```python
from build123d import *

# Parameters (mm, degrees)
SKETCH1_W           = 165
SKETCH1_H           = 81
SKETCH1_W_2         = 74
SKETCH1_H_2         = 50
BOSS_EXTRUDE1_DEPTH = 6
SKETCH2_W           = 108
SKETCH2_H           = 68
SKETCH2_W_2         = 98.5
SKETCH2_H_2         = 58.5
BOSS_EXTRUDE2_DEPTH = 9


with BuildPart() as part:
    # Sketch1 → Boss-Extrude1 (new body)
    with BuildSketch(Plane.XY):
        Rectangle(SKETCH1_W, SKETCH1_H)
        Rectangle(SKETCH1_W_2, SKETCH1_H_2, mode=Mode.SUBTRACT)
    extrude(amount=BOSS_EXTRUDE1_DEPTH)

    # Sketch2 → Boss-Extrude2 (add)
    with BuildSketch(Plane.XY):
        Rectangle(SKETCH2_W, SKETCH2_H)
        Rectangle(SKETCH2_W_2, SKETCH2_H_2, mode=Mode.SUBTRACT)
    extrude(amount=BOSS_EXTRUDE2_DEPTH)


solid = part.part
```
The listing builds one solid part. Answer for the finished solid, in the listing's coordinates (mm). A direction names the side the tool comes from. Give positions to 0.01 mm unless a question says otherwise; leave off trailing zeros. Order: outer loops, then holes, each group sorted by start corner. A loop starts at its lowest first (then second) coordinate and runs counter-clockwise, first axis right, second up. Notation, with made-up numbers: (-11, -3) -> (17, -3) arc R18 ccw to (17, 5) -> close; hole circle Ø6 at (-23.75, -12.75). An arc over 180 degrees is marked (long way). Answer as a JSON object with one key per item and string values. Group by question number.
Item 1: A tool of negligible diameter and unlimited length cuts with its end or side. For faces 4 (the flat face through (-1, -34, 7)), 5 (the flat face through (-54, 0, 7)), 6 (the flat face through (-1, 34, 7)), 7 (the flat face through (-49.25, 0, 7)), 8 (the flat face through (54, 0, 7)), from which of +Z, -Z, +X, -X, +Y, -Y can it reach the whole face along a straight path? Write none if from no direction.
Item 2: Consider L1, parallel to X at y = 13.5, z = 7; L2, parallel to X at y = 9, z = 1; L3, parallel to Y at x = 5.5, z = 7.5. Determine where each line is inside the solid, lowest interval first. Write a range as from..to.
Item 3: The part is cut by section A-A on y = 0. Write down the section's boundary in (x, z).
Item 4: Flat-ended cylindrical pins translate along their axes: pin 1 (1.5 mm diameter, centred on x = -19, z = 8, fed in from -Y); pin 2 (2.5 mm diameter, centred on x = -26.5, z = 8, fed in from +Y); pin 3 (3.5 mm diameter, centred on y = 5.5, z = 8, fed in from +X). Find the tip coordinate at first contact, or state that the pin passes through.
Item 5: The part is cut by section C-C on x = -27. Write down the section's boundary in (y, z).
Item 6: The part is cut by section D-D on y = 26.5. Write down the section's boundary in (x, z).
Item 7: The part is cut by section B-B on z = 2.5. Write down the section's boundary in (x, y).
Item 8: Determine the mould class of faces 1 (the flat face through (82.5, -1, 3)), 2 (the flat face through (-37, 0, 3)), 3 (the flat face through (-1, -40.5, 3)) for opening direction Y: pulls with the +Y half, pulls with the -Y half, needs draft (parallel to the pull), parting line crosses it, or undercut.
Result set:
{
 "1": {"face 4": "+Z, +X, -X, -Y", "face 5": "+Z, -X, +Y, -Y", "face 6": "+Z, +X, -X, +Y", "face 7": "+Z", "face 8": "+Z, +X, +Y, -Y"},
 "2": {"L1": "-54..-49.25, 49.25..54", "L2": "-82.5..-37, 37..82.5", "L3": "-34..-29.25, 29.25..34"},
 "3": {"outline": "(-82.5, 0) -> (-37, 0) -> (-37, 6) -> (-49.25, 6) -> (-49.25, 9) -> (-54, 9) -> (-54, 6) -> (-82.5, 6) -> close; (37, 0) -> (82.5, 0) -> (82.5, 6) -> (54, 6) -> (54, 9) -> (49.25, 9) -> (49.25, 6) -> (37, 6) -> close"},
 "4": {"pin 1": "y = -34", "pin 2": "y = 34", "pin 3": "x = 54"},
 "5": {"outline": "(-40.5, 0) -> (-25, 0) -> (-25, 6) -> (-29.25, 6) -> (-29.25, 9) -> (-34, 9) -> (-34, 6) -> (-40.5, 6) -> close; (25, 0) -> (40.5, 0) -> (40.5, 6) -> (34, 6) -> (34, 9) -> (29.25, 9) -> (29.25, 6) -> (25, 6) -> close"},
 "6": {"outline": "(-82.5, 0) -> (82.5, 0) -> (82.5, 6) -> (54, 6) -> (54, 9) -> (49.25, 9) -> (49.25, 6) -> (-49.25, 6) -> (-49.25, 9) -> (-54, 9) -> (-54, 6) -> (-82.5, 6) -> close"},
 "7": {"outline": "(-82.5, -40.5) -> (82.5, -40.5) -> (82.5, 40.5) -> (-82.5, 40.5) -> close; hole (-37, -25) -> (37, -25) -> (37, 25) -> (-37, 25) -> close"},
 "8": {"face 1": "needs draft", "face 2": "undercut", "face 3": "pulls with the -Y half"}
}
